Verification items for the finished model (mm, model axes). Give positions to 0.01 mm unless a question says otherwise; leave off trailing zeros. Order: outer loops, then holes, each group sorted by start corner. A loop starts at its lowest first (then second) coordinate and runs counter-clockwise, first axis right, second up. Notation, with made-up numbers: (9, 64.5) - (27, 64.5) arc R24 cw to (27, 87.5) - close; hole circle Ø10 at (10, 26). An arc over 180 degrees is marked (long way). Answer as a JSON object with one key per item and string values.
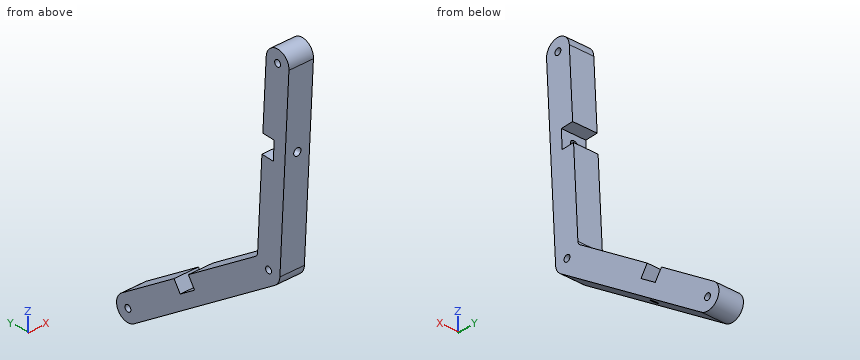
```python
from build123d import *

# Parameters (mm, degrees)
BOSS_EXTRUDE1_DEPTH        = 12.7
CUT_EXTRUDE1_DEPTH         = 132.57770374
AXEL_HOLES_D               = 3.2639
MOUNTING_HOLES_D           = 3.7973
MOUNTING_HOLES_ON_FACE_2_D = 3.7973
FILLET1_R                  = 2.54


with BuildPart() as part:
    # Sketch1 → Boss-Extrude1 (new body)
    with BuildSketch(Plane(origin=(0, 0, 0), x_dir=(0, 0, -1), z_dir=(1, 0, 0))):
        with BuildLine():
            Line((-93.814317406, 1.29451642), (-3.560533752, 6.167025361))
            Line((-3.560533752, 6.167025361), (45.786074597, 81.892840322))
            ThreePointArc((45.786074597, 81.892840322), (54.573019473, 83.746107639), (56.42628679, 74.959162763))
            Line((56.42628679, 74.959162763), (5.320106096, -3.46683878))
            ThreePointArc((5.320106096, -3.46683878), (3.175, -5.499261314), (0.342317406, -6.34076642))
            Line((0.342317406, -6.34076642), (-93.129682594, -11.38701642))
            ThreePointArc((-93.129682594, -11.38701642), (-99.81276642, -5.388567406), (-93.814317406, 1.29451642))
        make_face()
    extrude(amount=BOSS_EXTRUDE1_DEPTH)

    # Sketch2 → Cut-Extrude1 (cut, through all)
    with BuildSketch(Plane(origin=(12.7, 0, 0), x_dir=(0, 0, -1), z_dir=(1, 0, 0))):
        Polygon((-59.042239928, 3.171748061), (-58.699922522, -3.169018359), (-49.188772892, -2.65554225), (-49.531090298, 3.68522417), align=None)
        Polygon((21.574047399, 44.73779456), (26.894153496, 41.270955781), (32.094411665, 49.251114925), (26.774305568, 52.717953705), align=None)
    extrude(amount=-CUT_EXTRUDE1_DEPTH, mode=Mode.SUBTRACT)

    # Axel Holes (through all)
    with Locations(Plane(origin=(12.7, -5.04625, 93.472), x_dir=(0, 0, 1), z_dir=(1, 0, 0))):
        with Locations((0, 0), (-93.472, -5.04625), (-144.578180694, -83.472251543)):
            Hole(AXEL_HOLES_D / 2)

    # Mounting Holes (through all)
    with Locations(Plane(origin=(6.35, -2.912280304, 53.944347707), x_dir=(0, -0.053908252869, 0.998545892923), z_dir=(0, 0.998545892923, 0.053908252869))):
        with Locations((0, 0)):
            Hole(MOUNTING_HOLES_D / 2)

    # Mounting Holes on face 2 (through all)
    with Locations(Plane(origin=(6.35, 45.261035353, -29.49428258), x_dir=(0, 0.837811925843, -0.545958951676), z_dir=(0, 0.545958951676, 0.837811925843))):
        with Locations((0, 0)):
            Hole(MOUNTING_HOLES_ON_FACE_2_D / 2)

    # Fillet1
    fillet1_edges = [part.edges().sort_by_distance(p)[0] for p in [
        (6.35, 6.167025361, 3.560533752),
    ]]
    fillet(fillet1_edges, radius=FILLET1_R)


solid = part.part
```
(1) Material ranges on line 1 along Y through (x, z) = (5.5, 0); line 2 along Y through (x, z) = (6.25, 21); line 3 along Y through (x, z) = (1.25, -37.5), recorded low to high. Write a range as [from, to].
Computed values:
{"line 1": "y = [-6.36, -1.63], [1.63, 11.63]", "line 2": "y = [-7.49, 5.23]", "line 3": "y = [45.92, 69.18]"}
(2) Section check B-B (y = 24). Record the cut outline in (x, z), then the cut area to 3 significant figures.
Computed values:
{"outline": "(0, -23.22) - (12.7, -23.22) - (12.7, -8.06) - (0, -8.06) - close", "area": "193 mm²"}
(3) Gauge pin test, flat ends, axial feed: pin 1 Ø1 at (x, y) = (10.5, 40) entering from -Z; pin 2 Ø12 at (y, z) = (3.5, 61) entering from -X; pin 3 Ø1.5 at (x, z) = (3, -21) entering from +Y; pin 4 Ø3 at (x, z) = (10.5, -40.5) entering from -Y. Record the tip position at first contact, or that the pin passes through.
Computed values:
{"pin 1": "stops at z = -33.97", "pin 2": "stops at x = 0", "pin 3": "stops at y = 44.74", "pin 4": "stops at y = 48.22"}
(4) Section check C-C (z = -41). Record the cut outline in (x, y).
Computed values:
{"outline": "(0, 51.29) - (12.7, 51.29) - (12.7, 74.55) - (0, 74.55) - close"}
(5) Section check A-A (x = 10). Record the cut outline in (y, z), then the cut area to 3 significant figures.
Computed values:
{"outline": "(-11.39, 93.13) - (-6.34, -0.34) arc R6.35 ccw to (-3.47, -5.32) - (74.96, -56.43) arc R6.35 ccw to (81.89, -45.79) - (52.72, -26.77) - (49.25, -32.09) - (41.27, -26.89) - (44.74, -21.57) - (7.25, 2.86) arc R2.54 cw to (6.1, 4.85) - (3.69, 49.53) - (-2.66, 49.19) - (-3.17, 58.7) - (3.17, 59.04) - (1.29, 93.81) arc R6.35 ccw to start; hole circle Ø3.26 at (-5.05, 93.47); hole circle Ø3.26 at (0, 0); hole circle Ø3.26 at (78.43, -51.11)", "area": "2,360 mm²"}
